Autodesk Inventor part; units mm, degrees
ref_plane "YZ Plane" through (0, 0, 0) normal (1, 0, 0) x (0, 1, 0)
ref_plane "XZ Plane" through (0, 0, 0) normal (0, 1, 0) x (-1, 0, 0)
ref_plane "XY Plane" through (0, 0, 0) normal (0, 0, 1) x (1, 0, 0)
sketch "Boceto1" plane through (0, 0, 0) normal (0, 0, 1) x (1, 0, 0)
  line L0 (0, 0) -> (40, 0)
  line L1 (40, 0) -> (40, 60)
  line L2 (40, 60) -> (0, 60)
  line L3 (0, 60) -> (0, 0)
  circle A0 centre (20, 32) radius 4
  dimension "d0" = 40
  dimension "d1" = 60
  dimension "d2" = 8
  dimension "d31" = 32
extrude "Extrusión1" add sketch "Boceto1" along normal blind 10
sketch "Boceto2" plane through (0, 0, 10) normal (0, 0, 1) x (1, 0, 0)
  circle A0 centre (20, 32) radius 4
  circle A1 centre (20, 32) radius 12.59
  point P0 (0, 0)
  dimension "d5" = 25.18
extrude "Extrusión2" cut sketch "Boceto2" against normal blind 8
fillet "Empalme1" radius 8 2 edges at (40, 60, 5) (0, 60, 5)
sketch "Boceto4" plane through (0, 0, 0) normal (0, 0, -1) x (-1, 0, 0)
  circle A0 centre (-20, 40.5) radius 1.5
  circle A1 centre (-20, 23.5) radius 1.5
  circle A2 centre (-20, 32) radius 4
  point P0 (0, 0)
  dimension "d11" = 3
  dimension "d12" = 3
  dimension "d14" = 8.5
  dimension "d15" = 17
extrude "Extrusión4" cut sketch "Boceto4" against normal blind 2 contours A0 | A1
sketch "Boceto5" plane through (0, 0, 10) normal (0, 0, 1) x (1, 0, 0)
  line L0 (0, 52) -> (0, 0)
  line L1 (0, 0) -> (15, 0)
  line L2 (15, 0) -> (15, 10)
  line L3 (15, 10) -> (0, 10)
  line L4 (0, 10) -> (0, 0)
  line L5 (40, 0) -> (40, 52)
  line L6 (40, 0) -> (25, 0)
  line L7 (25, 0) -> (25, 10)
  line L8 (25, 10) -> (40, 10)
  line L9 (40, 10) -> (40, 0)
  point P0 (0, 10)
  dimension "d18" = 15
  dimension "d19" = 10
  dimension "d20" = 15
  dimension "d21" = 10
extrude "Extrusión5" add sketch "Boceto5" along normal blind 15
sketch "Boceto6" plane through (0, 10, 10) normal (0, 1, 0) x (1, 0, 0)
  line L0 (15, -15) -> (0, -15)
  line L1 (0, 0) -> (15, 0)
  line L2 (15, 0) -> (15, -15)
  circle A0 centre (7.5, -7.5) radius 3
  line L3 (25, -15) -> (40, -15)
  circle A1 centre (32.5, -7.5) radius 3
  circle A2 centre (7.5, -7.5) radius 4.25
  circle A3 centre (32.5, -7.5) radius 4.25
  line L4 (0, 0) -> (0, -15)
  line L5 (40, 0) -> (40, -15)
  line L6 (40, 0) -> (32, 0)
  point P0 (0, 10)
  point P1 (40, -7.5)
  dimension "d24" = 6
  dimension "d25" = 6
  dimension "d32" = 8.5
  dimension "d33" = 8.5
  dimension "d36" = 7.5
  dimension "d37" = 7.5
  dimension "d38" = 7.5
  dimension "d39" = 7.5
extrude "Extrusión6" cut sketch "Boceto6" against normal blind 5 contours A0 | A1
extrude "Extrusión7" cut sketch "Boceto6" against normal blind 5 contours A2 | A3
sketch "Boceto7" plane through (0, 0, 0) normal (0, -1, 0) x (1, 0, 0)
  circle A0 centre (32.5, 17.5) radius 4.25
  circle A1 centre (32.5, 17.5) radius 3
  circle A2 centre (7.5, 17.5) radius 4.25
  circle A3 centre (7.5, 17.5) radius 3
  point P0 (0, 0)
  dimension "d40" = 6
  dimension "d41" = 6
extrude "Extrusión8" cut sketch "Boceto7" against normal blind 5 contours A1 | A3
fillet "Empalme2" radius 2 1 edges at (7.5, 10, 10)
fillet "Empalme3" radius 2 1 edges at (32.5, 10, 10)
properties part number "sujeción motor-acople"
The model under review builds one solid part; all positions refer to its coordinate system, in mm. A direction names the side the tool comes from. Coordinates: 2 decimals unless noted, no trailing zeros. Order: outer loops, then holes, each group sorted by start corner. A loop starts at its lowest first (then second) coordinate and runs counter-clockwise, first axis right, second up. Notation, with made-up numbers: (42, 47) -> (70, 47) arc R19 cw to (70, 76) -> close; hole circle Ø6 at (71.25, 35). An arc over 180 degrees is marked (long way). Answer in a Markdown table with one row per item. Add a question column.
Item 1: We need section D-D on y = 40.5. Write out the cut boundary in (x, z).
Item 2: Clearance check with flat-ended pins moving along their axes: pin 1 (3.5 mm diameter, centred on x = 32.5, z = 17.5, fed in from -Y); pin 2 (10 mm diameter, centred on x = 14.5, y = 29.5, fed in from +Z); pin 3 (6.5 mm diameter, centred on x = 9.5, z = 17.5, fed in from +Y); pin 4 (4 mm diameter, centred on x = 33.5, z = 16.5, fed in from +Y). State where each tip first meets the part, or that it passes through.
Item 3: We need section A-A on z = 17.5. Write out the cut boundary in (x, y).
Item 4: We need section C-C on z = 9. Write out the cut boundary in (x, y).
Item 5: Machinability: for faces 1 (the flat face through (15, 5, 17)), 2 (the flat face through (19.7, 0, 9.5)), 3 (the flat face through (17, 35, 2)), 4 (the flat face through (0, 21, 7)), 5 (the cylindrical face through (6.58, 7.54, 21.65)), which of the approach directions +Z, -Z, +X, -X, +Y, -Y give a long, thin tool a straight path to every point of the face, cutting with its end or side? Answer none if there is none.
Item 6: Mouldability with a two-part tool opening along Z and no side actions: class faces 6 (the cylindrical face through (17.27, 19.71, 6.06)), 7 (the flat face through (34.3, 5, 20.3)), 8 (the flat face through (7, 5, 25)) as +Z half, -Z half, draft (parallel to the pull), parting line (faces both ways), or undercut.
Item 7: We need section B-B on x = 20. Write out the cut boundary in (y, z), plus the area to 3 significant figures.
Item 8: To check wall thickness, follow probe 1 along Y at (x, z) = (20, 0.45); probe 2 along Z at (x, y) = (7.5, 8.25); probe 3 along X at (y, z) = (6.6, 17.5). State the ranges of each line that lie inside material, in increasing order.
Final values:
| question | item | result |
|---|---|---|
| 1 | outline | (0, 0) -> (18.5, 0) -> (18.5, 2) -> (10.71, 2) -> (10.71, 10) -> (0, 10) -> close; (21.5, 0) -> (40, 0) -> (40, 10) -> (29.29, 10) -> (29.29, 2) -> (21.5, 2) -> close |
| 2 | pin 1 | passes through |
| 2 | pin 2 | stops at z = 2 |
| 2 | pin 3 | stops at y = 10 |
| 2 | pin 4 | stops at y = 5 |
| 3 | outline | (0, 0) -> (4.5, 0) -> (4.5, 5) -> (3.25, 5) -> (3.25, 10) -> (0, 10) -> close; (10.5, 0) -> (15, 0) -> (15, 10) -> (11.75, 10) -> (11.75, 5) -> (10.5, 5) -> close; (25, 0) -> (29.5, 0) -> (29.5, 5) -> (28.25, 5) -> (28.25, 10) -> (25, 10) -> close; (35.5, 0) -> (40, 0) -> (40, 10) -> (36.75, 10) -> (36.75, 5) -> (35.5, 5) -> close |
| 4 | outline | (0, 0) -> (40, 0) -> (40, 52) arc R8 ccw to (32, 60) -> (8, 60) arc R8 ccw to (0, 52) -> close; hole circle Ø25.18 at (20, 32) |
| 5 | face 1 | +Z, +Y, -Y |
| 5 | face 2 | +Z, -Z, +X, -X, -Y |
| 5 | face 3 | +Z |
| 5 | face 4 | +Z, -Z, -X, +Y, -Y |
| 5 | face 5 | +Y |
| 6 | face 6 | draft |
| 6 | face 7 | undercut |
| 6 | face 8 | +Z half |
| 7 | outline | (0, 0) -> (22, 0) -> (22, 2) -> (19.41, 2) -> (19.41, 10) -> (0, 10) -> close; (25, 0) -> (28, 0) -> (28, 2) -> (25, 2) -> close; (36, 0) -> (39, 0) -> (39, 2) -> (36, 2) -> close; (42, 0) -> (60, 0) -> (60, 10) -> (44.59, 10) -> (44.59, 2) -> (42, 2) -> close |
| 7 | area | 371 mm2 |
| 8 | probe 1 | y = 0 to 22, 25 to 28, 36 to 39, 42 to 60 |
| 8 | probe 2 | z = 0 to 13.25, 21.75 to 25 |
| 8 | probe 3 | x = 0 to 3.25, 11.75 to 15, 25 to 28.25, 36.75 to 40 |
